Build history of the part. All positions in model axes, mm. A direction names the side the tool comes from. Give positions to 0.01 mm unless a question says otherwise; leave off trailing zeros. Order: outer loops, then holes, each group sorted by start corner. A loop starts at its lowest first (then second) coordinate and runs counter-clockwise, first axis right, second up. Notation, with made-up numbers: M 39,33.25 L 87,33.25 A19 ccw 87,56.25 Z; hole C 37,45 d1. An arc over 180 degrees is marked long. Answer as CSV lines item,"result".
from build123d import *

# Parameters (mm, degrees)
SKETCH1_W               = 101.6
SKETCH1_H               = 205.74
BATTERY_SIDE_DEPTH      = 107.95
SKETCH6_W               = 60.325
SKETCH6_H               = 1.5875
SKETCH6_W_2             = 52.3875
BATTERY_TAB_BASES_DEPTH = 9.525
SKETCH7_W               = 1.5875
SKETCH7_H               = 60.325
SKETCH7_H_2             = 52.3875
BATTERY_TABS_DEPTH      = 25.4
BATTERY_TAB_HOLES_REACH = 113.125
SKETCH8_R               = 3
SKETCH2_W               = 165.1
SKETCH2_H               = 205.74
MOTOR_SIDE_DEPTH        = 42.8625
SKETCH3_W               = 28.575
SKETCH3_H               = 1.5875
SKETCH3_W_2             = 25.4
MOTOR_TAB_BASES_DEPTH   = 57.15
SKETCH4_W               = 1.5875
SKETCH4_H               = 28.575
SKETCH4_H_2             = 25.4
MOTOR_TABS_DEPTH        = 15.875
MOTOR_TAB_HOLES_REACH   = 335.375
SKETCH5_R               = 3


with BuildPart() as part:
    # Sketch1 → Battery Side (new body)
    with BuildSketch(Plane(origin=(0, 0, 0), x_dir=(1, 0, 0), z_dir=(0, 1, 0))):
        with Locations((50.8, 102.87)):
            Rectangle(SKETCH1_W, SKETCH1_H)
    extrude(amount=BATTERY_SIDE_DEPTH)

    # Sketch6 → Battery Tab Bases (add)
    with BuildSketch(Plane.ZY):
        with Locations((-151.765, 38.89375)):
            Rectangle(SKETCH6_W, SKETCH6_H)
        with Locations((-63.65875, 38.89375)):
            Rectangle(SKETCH6_W_2, SKETCH6_H)
    extrude(amount=BATTERY_TAB_BASES_DEPTH)

    # Sketch7 → Battery Tabs (add)
    with BuildSketch(Plane(origin=(0, 39.6875, 0), x_dir=(1, 0, 0), z_dir=(0, 1, 0))):
        with Locations((-8.73125, 151.765)):
            Rectangle(SKETCH7_W, SKETCH7_H)
        with Locations((-8.73125, 63.65875)):
            Rectangle(SKETCH7_W, SKETCH7_H_2)
    extrude(amount=BATTERY_TABS_DEPTH)

    # Sketch8 → Battery Tab Holes (cut, up to next)
    with BuildSketch(Plane.ZY.offset(9.525), mode=Mode.PRIVATE) as battery_tab_holes_sk1:
        with Locations((-172.495098328, 50.0063)):
            Circle(SKETCH8_R)
    battery_tab_holes_tool1 = extrude(battery_tab_holes_sk1.sketch, amount=-BATTERY_TAB_HOLES_REACH, mode=Mode.PRIVATE) & part.part
    add(battery_tab_holes_tool1.solids().sort_by_distance((-9.525, 50.0063, -172.495098))[0], mode=Mode.SUBTRACT)
    # Sketch8 → Battery Tab Holes (cut, up to next)
    with BuildSketch(Plane.ZY.offset(9.525), mode=Mode.PRIVATE) as battery_tab_holes_sk2:
        with Locations((-55.26378475, 50.0063)):
            Circle(SKETCH8_R)
    battery_tab_holes_tool2 = extrude(battery_tab_holes_sk2.sketch, amount=-BATTERY_TAB_HOLES_REACH, mode=Mode.PRIVATE) & part.part
    add(battery_tab_holes_tool2.solids().sort_by_distance((-9.525, 50.0063, -55.263785))[0], mode=Mode.SUBTRACT)

    # Sketch2 → Motor Side (add)
    with BuildSketch(Plane(origin=(0, 0, 0), x_dir=(1, 0, 0), z_dir=(0, 1, 0))):
        with Locations((184.15, 102.87)):
            Rectangle(SKETCH2_W, SKETCH2_H)
    extrude(amount=MOTOR_SIDE_DEPTH)

    # Sketch3 → Motor Tab Bases (add)
    with BuildSketch(Plane(origin=(266.7, 0, 0), x_dir=(0, 0, -1), z_dir=(1, 0, 0))):
        with Locations((39.6875, 42.06875)):
            Rectangle(SKETCH3_W, SKETCH3_H)
        with Locations((107.95, 42.06875)):
            Rectangle(SKETCH3_W, SKETCH3_H)
        with Locations((163.5125, 42.06875)):
            Rectangle(SKETCH3_W_2, SKETCH3_H)
    extrude(amount=MOTOR_TAB_BASES_DEPTH)

    # Sketch4 → Motor Tabs (add)
    with BuildSketch(Plane(origin=(0, 42.8625, 0), x_dir=(1, 0, 0), z_dir=(0, 1, 0))):
        with Locations((323.05625, 39.6875)):
            Rectangle(SKETCH4_W, SKETCH4_H)
        with Locations((323.05625, 107.95)):
            Rectangle(SKETCH4_W, SKETCH4_H)
        with Locations((323.05625, 163.5125)):
            Rectangle(SKETCH4_W, SKETCH4_H_2)
    extrude(amount=MOTOR_TABS_DEPTH)

    # Sketch5 → Motor Tab Holes (cut, up to next)
    with BuildSketch(Plane(origin=(323.85, 0, 0), x_dir=(0, 0, -1), z_dir=(1, 0, 0)), mode=Mode.PRIVATE) as motor_tab_holes_sk1:
        with Locations((33.3375, 50.00625)):
            Circle(SKETCH5_R)
    motor_tab_holes_tool1 = extrude(motor_tab_holes_sk1.sketch, amount=-MOTOR_TAB_HOLES_REACH, mode=Mode.PRIVATE) & part.part
    add(motor_tab_holes_tool1.solids().sort_by_distance((323.85, 50.00625, -33.3375))[0], mode=Mode.SUBTRACT)
    # Sketch5 → Motor Tab Holes (cut, up to next)
    with BuildSketch(Plane(origin=(323.85, 0, 0), x_dir=(0, 0, -1), z_dir=(1, 0, 0)), mode=Mode.PRIVATE) as motor_tab_holes_sk2:
        with Locations((46.0375, 50.00625)):
            Circle(SKETCH5_R)
    motor_tab_holes_tool2 = extrude(motor_tab_holes_sk2.sketch, amount=-MOTOR_TAB_HOLES_REACH, mode=Mode.PRIVATE) & part.part
    add(motor_tab_holes_tool2.solids().sort_by_distance((323.85, 50.00625, -46.0375))[0], mode=Mode.SUBTRACT)
    # Sketch5 → Motor Tab Holes (cut, up to next)
    with BuildSketch(Plane(origin=(323.85, 0, 0), x_dir=(0, 0, -1), z_dir=(1, 0, 0)), mode=Mode.PRIVATE) as motor_tab_holes_sk3:
        with Locations((101.6, 50.00625)):
            Circle(SKETCH5_R)
    motor_tab_holes_tool3 = extrude(motor_tab_holes_sk3.sketch, amount=-MOTOR_TAB_HOLES_REACH, mode=Mode.PRIVATE) & part.part
    add(motor_tab_holes_tool3.solids().sort_by_distance((323.85, 50.00625, -101.6))[0], mode=Mode.SUBTRACT)
    # Sketch5 → Motor Tab Holes (cut, up to next)
    with BuildSketch(Plane(origin=(323.85, 0, 0), x_dir=(0, 0, -1), z_dir=(1, 0, 0)), mode=Mode.PRIVATE) as motor_tab_holes_sk4:
        with Locations((114.3, 50.00625)):
            Circle(SKETCH5_R)
    motor_tab_holes_tool4 = extrude(motor_tab_holes_sk4.sketch, amount=-MOTOR_TAB_HOLES_REACH, mode=Mode.PRIVATE) & part.part
    add(motor_tab_holes_tool4.solids().sort_by_distance((323.85, 50.00625, -114.3))[0], mode=Mode.SUBTRACT)
    # Sketch5 → Motor Tab Holes (cut, up to next)
    with BuildSketch(Plane(origin=(323.85, 0, 0), x_dir=(0, 0, -1), z_dir=(1, 0, 0)), mode=Mode.PRIVATE) as motor_tab_holes_sk5:
        with Locations((158.75, 50.00625)):
            Circle(SKETCH5_R)
    motor_tab_holes_tool5 = extrude(motor_tab_holes_sk5.sketch, amount=-MOTOR_TAB_HOLES_REACH, mode=Mode.PRIVATE) & part.part
    add(motor_tab_holes_tool5.solids().sort_by_distance((323.85, 50.00625, -158.75))[0], mode=Mode.SUBTRACT)


solid = part.part
Item 1: Drop flat-ended pins along their axis: pin 1 (1 mm diameter, centred on y = 89, z = -110, fed in from +X); pin 2 (14 mm diameter, centred on x = 303, y = 51.5, fed in from -Z); pin 3 (8.5 mm diameter, centred on x = 287, y = 46, fed in from +Z); pin 4 (1.7 mm diameter, centred on x = 322.5, z = -102, fed in from +Y). Give the stop position or say it passes through.
Geometry says:
pin 1,"stops at x = 101.6"
pin 2,"passes through"
pin 3,"stops at z = -25.4"
pin 4,"stops at y = 58.74"
Item 2: 3-axis set-ups, long thin cutter, end or side, ignore diameter. For faces 4 (the flat face through (-8.3, 47.5, -89.852)), 5 (the flat face through (322.262, 51, -163)), 6 (the flat face through (301, 42, -25.4)), 7 (the flat face through (301, 42, -93.663)), 8 (the flat face through (-8.3, 47.5, -181.927)): which of +Z, -Z, +X, -X, +Y, -Y reach the whole face in a straight line?
Geometry says:
face 4,"-X, +Y, -Y"
face 5,"+Z, -Z, +Y"
face 6,"+Z, +X, +Y, -Y"
face 7,"+X, +Y, -Y"
face 8,"-Z, -X, +Y, -Y"
Item 3: Band-saw the part on B-B (x = 142). Give the cut face in (y, z), and give its area (3 significant figures).
Geometry says:
outline,"M 0,-205.74 L 42.86,-205.74 L 42.86,0 L 0,0 Z"
area,"8,820 mm2"
Item 4: Probe line 1 along X through (y, z) = (41, -128) (1 decimal); line 2 along X through (y, z) = (78, -156); line 3 along Y through (x, z) = (208.5, -81). List the from-to ranges inside material, lowest first. Write a range as from..to.
Geometry says:
line 1,"x = -9.5..-7.9, 0..266.7"
line 2,"x = 0..101.6"
line 3,"y = 0..42.86"
Item 5: Band-saw the part on C-C (y = 100). Give the cut face in (x, z), and give its area (3 significant figures).
Geometry says:
outline,"M 0,-205.74 L 101.6,-205.74 L 101.6,0 L 0,0 Z"
area,"20,900 mm2"
Item 6: Pull direction X, two halves, no side cores. Call faces 1 (the flat face through (323.85, 50, -163)), 2 (the flat face through (-7.937, 52, -63)), 3 (the flat face through (-5, 38.1, -64)): released by +X, released by -X, zero draft, split by the parting line, or undercut.
Geometry says:
face 1,"released by +X"
face 2,"undercut"
face 3,"zero draft"
